from build123d import *

# Parameters (mm, degrees)
F0_R     = 2.54
F1_DEPTH = 5.08


with BuildPart() as f1:
    # F0 (on Front) → F1 (new body)
    with BuildSketch(Plane.XZ):
        with BuildLine():
            ThreePointArc((-42.2490756804, -10.6206300524), (-40.2114050241, -8.3410427676), (-39.4752932215, -5.3734243105))
            ThreePointArc((-39.4752932215, -5.3734243105), (-42.8576747645, 0.2404638869), (-49.4015107627, -0.1262185685))
            ThreePointArc((-49.4015107627, -0.1262185685), (-51.0724989635, -8.9496418517), (-42.2490756804, -10.6206300524))
        make_face()
        with Locations((-45.8252932215, -5.3734243105)):
            Circle(F0_R, mode=Mode.SUBTRACT)
        with BuildLine():
            ThreePointArc((-49.4015107627, -0.1262185685), (-42.8576747645, 0.2404638869), (-39.4752932215, -5.3734243105))
            ThreePointArc((-39.4752932215, -5.3734243105), (-40.2114050241, -8.3410427676), (-42.2490756804, -10.6206300524))
            Line((-42.2490756804, -10.6206300524), (62.6950390311, 60.9037206843))
            ThreePointArc((62.6950390311, 60.9037206843), (53.8716158307, 62.5747090371), (55.5426040793, 71.3981322572))
            Line((55.5426040793, 71.3981322572), (-49.4015107627, -0.1262185685))
        make_face()
        with BuildLine():
            Line((129.0034844631, 121.4651778314), (55.5426040793, 71.3981322572))
            ThreePointArc((55.5426040793, 71.3981322572), (62.086440076, 71.7648147095), (65.4688216172, 66.150926513))
            ThreePointArc((65.4688216172, 66.150926513), (64.7327097786, 63.1833079879), (62.6950390311, 60.9037206843))
            Line((62.6950390311, 60.9037206843), (136.1559195454, 110.9707663475))
            ThreePointArc((136.1559195454, 110.9707663475), (127.3324962623, 112.6417545483), (129.0034844631, 121.4651778314))
        make_face()
        with BuildLine():
            ThreePointArc((65.4688216172, 66.150926513), (62.086440076, 71.7648147095), (55.5426040793, 71.3981322572))
            ThreePointArc((55.5426040793, 71.3981322572), (53.8716158307, 62.5747090371), (62.6950390311, 60.9037206843))
            ThreePointArc((62.6950390311, 60.9037206843), (64.7327097786, 63.1833079879), (65.4688216172, 66.150926513))
        make_face()
        with Locations((59.1188216172, 66.150926513)):
            Circle(F0_R, mode=Mode.SUBTRACT)
        with BuildLine():
            ThreePointArc((138.9297020042, 116.2179720895), (135.5473204613, 121.8318602869), (129.0034844631, 121.4651778314))
            ThreePointArc((129.0034844631, 121.4651778314), (127.3324962623, 112.6417545483), (136.1559195454, 110.9707663475))
            ThreePointArc((136.1559195454, 110.9707663475), (138.1935902017, 113.2503536324), (138.9297020042, 116.2179720895))
        make_face()
        with Locations((132.5797020042, 116.2179720895)):
            Circle(F0_R, mode=Mode.SUBTRACT)
    extrude(amount=F1_DEPTH)


solid = f1.part
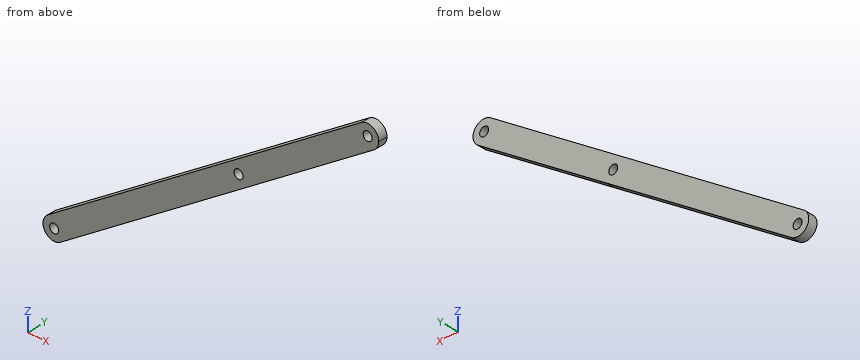
Design review of the part built by this model. Coordinates are the model's own, in mm. Coordinates: 2 decimals unless noted, no trailing zeros. Order: outer loops, then holes, each group sorted by start corner. A loop starts at its lowest first (then second) coordinate and runs counter-clockwise, first axis right, second up.
Item 1: Take a section at A-A, the plane y = -1.4. Write out the cut boundary in (x, z), then the cut area to 3 significant figures.
Item 2: For pin 1 Ø3 at (x, y) = (82.5, -3) entering from +Z; pin 2 Ø2 at (y, z) = (-1, 106) entering from +X; pin 3 Ø1 at (x, y) = (52, -3.5) entering from +Z, all flat-tipped, find the tip position at first contact; note any pin that passes through.
Item 3: Take a section at B-B, the plane z = 82. Write out the cut boundary in (x, y).
Item 4: Take a section at C-C, the plane x = 25. Write out the cut boundary in (y, z).
Item 5: For line 1 (Z direction, x = 57.5, y = -4.7); line 2 (X direction, y = -1.75, z = 67); line 3 (X direction, y = -0.5, z = 115), list the stretches that pass through material, from the lowest coordinate up.
The answers:
1. outline: (-49.4, -0.13) arc R6.35 ccw to (-42.25, -10.62) - (136.16, 110.97) arc R6.35 ccw to (129, 121.47) - close; hole circle Ø5.08 at (-45.83, -5.37); hole circle Ø5.08 at (59.12, 66.15); hole circle Ø5.08 at (132.58, 116.22)
1. area: 2,810 mm2
2. pin 1: stops at z = 90.79
2. pin 2: stops at x = 130.33
2. pin 3: stops at z = 69.32
3. outline: (71.1, -5.08) - (93.65, -5.08) - (93.65, 0) - (71.1, 0) - close
4. outline: (-5.08, 35.21) - (0, 35.21) - (0, 50.58) - (-5.08, 50.58) - close
5. line 1: z = 57.36 to 64.19, 68.11 to 72.73
5. line 2: x = 49.09 to 56.72, 61.51 to 71.64
5. line 3: x = 119.52 to 130.35, 134.81 to 138.81
